Could you check a few things on this model? Use its own coordinates, in mm. A direction names the side the tool comes from. Give positions to 0.01 mm unless a question says otherwise; leave off trailing zeros. Order: outer loops, then holes, each group sorted by start corner. A loop starts at its lowest first (then second) coordinate and runs counter-clockwise, first axis right, second up. Notation, with made-up numbers: M -15.5,78.5 L 10.5,78.5 A9 ccw 10.5,94.5 Z; hole C -1.75,18.5 d7. An arc over 180 degrees is marked long. Use a Markdown table: item, result. Add a question column.
Item 1: Suppose I cut it at A-A on y = 5. Count the separate pieces of the cut face and the enclosed holes in it, plus the area to 3 significant figures.
Item 2: I'm going to push flat-ended pins straight in: pin 1 Ø1.9 at (x, y) = (20, 5) entering from -Z; pin 2 Ø3.5 at (x, y) = (20, 5) entering from +Z; pin 3 Ø3 at (y, z) = (12.5, 1.5) entering from +X; pin 4 Ø0.9 at (y, z) = (13.5, 1.5) entering from +X. Where does each tip first touch, or does it pass through?
Item 3: Suppose I cut it at B-B on x = 5. Write out the boundary of the cut face in (y, z), plus the area to 3 significant figures.
Item 4: If we mould it in two halves opening along X, with no side actions, what happens to faces 6 (the face through (1.141, 1.203, 2.524)), 7 (the face through (30, 5, 2)), 8 (the face through (5, 25, 2)), 9 (the face through (11.384, 2.338, 4.187))? For each: released by +X, released by -X, zero draft, split by the parting line, or undercut.
Item 5: If I drill on L1, parallel to X at y = 16.25, z = 3.4; L2, parallel to Y at x = 7.5, z = 3; L3, parallel to Y at x = 10, z = 3.9, over which ranges is the centre line in solid material (lowest first)? Write a range as from..to.
Item 6: Suppose I cut it at C-C on z = 1.75. Write out the boundary of the cut face in (x, y), plus the area to 3 significant figures.
Item 7: For faces 1 (the face through (22.5, 14, 2)), 2 (the face through (0.23, 5.77, 4.76)), 3 (the face through (21.3, 3.7, 3.35)), 4 (the face through (-3, 10, 2)), 5 (the face through (25.51, 9.77, 4.76)), which set-ups out of +Z, -Z, +X, -X, +Y, -Y let a thin tool reach every point of the face, with its end or its side?
from build123d import *

# Parameters (mm, degrees)
SKETCH2_W                       = 15
SKETCH2_H                       = 15
BOSS_EXTRUDE1_DEPTH             = 5
M3_CLEARANCE_HOLE1_OUTLINE_R    = 1.6
M3_CLEARANCE_HOLE1_DEPTH        = 5
CBORE_FOR_M3_SBHCS1_D           = 3.2
CBORE_FOR_M3_SBHCS1_CBORE_D     = 6
CBORE_FOR_M3_SBHCS1_CBORE_DEPTH = 1.65
CHAMFER1_SIZE                   = 8
FILLET1_R                       = 4
FILLET2_R                       = 2.5
FILLET3_R                       = 0.8


# Read off the part's stored shape, not the designer's step: M3 Clearance Hole1
with BuildPart() as part:
    # Sketch2 → Boss-Extrude1 (new body)
    with BuildSketch(Plane.XY):
        Polygon((0, 10), (0, 0), (30, 0), (30, 10), (22.5, 10), (7.5, 10), align=None)
        Polygon((-7.5, 10), (0, 10), (7.5, 10), (7.5, 25), (-7.5, 25), align=None)
        with Locations((15, 17.5)):
            Rectangle(SKETCH2_W, SKETCH2_H)
    extrude(amount=BOSS_EXTRUDE1_DEPTH)

    # M3 Clearance Hole1 outline → M3 Clearance Hole1 (cut)
    with BuildSketch(Plane.XY):
        with Locations((7.5, 17.5)):
            Circle(M3_CLEARANCE_HOLE1_OUTLINE_R)
        with Locations((-2.5, 17.5)):
            Circle(M3_CLEARANCE_HOLE1_OUTLINE_R)
        with Locations((25, 5)):
            Circle(M3_CLEARANCE_HOLE1_OUTLINE_R)
        with Locations((5, 5)):
            Circle(M3_CLEARANCE_HOLE1_OUTLINE_R)
    extrude(amount=M3_CLEARANCE_HOLE1_DEPTH, mode=Mode.SUBTRACT)

    # CBORE for M3 SBHCS1 (through all)
    with Locations(Plane.XY.offset(5)):
        with Locations((20, 5), (10, 5)):
            CounterBoreHole(CBORE_FOR_M3_SBHCS1_D / 2, CBORE_FOR_M3_SBHCS1_CBORE_D / 2, CBORE_FOR_M3_SBHCS1_CBORE_DEPTH)

    # Chamfer1
    chamfer1_edges = [part.edges().sort_by_distance(p)[0] for p in [
        (22.5, 25, 2.5),
    ]]
    chamfer(chamfer1_edges, length=CHAMFER1_SIZE)

    # Fillet1
    fillet1_edges = [part.edges().sort_by_distance(p)[0] for p in [
        (-7.5, 10, 2.5),
        (-7.5, 25, 2.5),
        (30, 10, 2.5),
        (30, 0, 2.5),
        (0, 0, 2.5),
        (14.5, 25, 2.5),
        (22.5, 17, 2.5),
    ]]
    fillet(fillet1_edges, radius=FILLET1_R)

    # Fillet2
    fillet2_edges = [part.edges().sort_by_distance(p)[0] for p in [
        (22.5, 10, 2.5),
        (0, 10, 2.5),
    ]]
    fillet(fillet2_edges, radius=FILLET2_R)

    # Fillet3
    fillet3_edges = [part.edges().sort_by_distance(p)[0] for p in [
        (14.37387948, 24.69551813, 5),
        (22.5, 13.921572875, 0),
        (22.5, 13.921572875, 5),
        (25.5, 10, 5),
        (25.5, 10, 0),
        (-3, 10, 5),
        (-3, 10, 0),
        (23.232233047, 10.732233047, 0),
        (23.232233047, 10.732233047, 5),
        (-0.732233047, 9.267766953, 0),
        (-0.732233047, 9.267766953, 5),
        (4.671572875, 25, 5),
        (4.671572875, 25, 0),
        (18.5, 21, 0),
        (30, 5, 0),
        (15, 0, 0),
        (0, 5.75, 0),
        (-7.5, 17.5, 0),
        (1.171572875, 1.171572875, 0),
        (28.828427125, 1.171572875, 0),
        (28.828427125, 8.828427125, 0),
        (-6.328427125, 11.171572875, 0),
        (-6.328427125, 23.828427125, 0),
        (22.19551813, 16.87387948, 0),
        (14.37387948, 24.69551813, 0),
        (18.5, 21, 5),
        (-7.5, 17.5, 5),
        (0, 5.75, 5),
        (15, 0, 5),
        (30, 5, 5),
        (1.171572875, 1.171572875, 5),
        (28.828427125, 1.171572875, 5),
        (28.828427125, 8.828427125, 5),
        (-6.328427125, 11.171572875, 5),
        (-6.328427125, 23.828427125, 5),
        (22.19551813, 16.87387948, 5),
    ]]
    fillet(fillet3_edges, radius=FILLET3_R)


solid = part.part
Findings below:
| question | item | result |
|---|---|---|
| 1 | separate pieces | 5 |
| 1 | enclosed holes | 0 |
| 1 | area | 76.2 mm^2 |
| 2 | pin 1 | passes through |
| 2 | pin 2 | stops at z = 3.35 |
| 2 | pin 3 | stops at x = 23 |
| 2 | pin 4 | stops at x = 22.5 |
| 3 | outline | M 0,0.8 A0.8 ccw 0.8,0 L 3.4,0 L 3.4,5 L 0.8,5 A0.8 ccw 0,4.2 Z; M 6.6,0 L 24.2,0 A0.8 ccw 25,0.8 L 25,4.2 A0.8 ccw 24.2,5 L 6.6,5 Z |
| 3 | area | 108 mm^2 |
| 4 | face 6 | released by -X |
| 4 | face 7 | released by +X |
| 4 | face 8 | zero draft |
| 4 | face 9 | undercut |
| 5 | L1 | x = -7.5..-3.5, -1.5..6.5, 8.5..22.4 |
| 5 | L2 | y = 0..15.9, 19.1..25 |
| 5 | L3 | y = 0..2, 8..25 |
| 6 | outline | M -7.5,14 A4 ccw -3.5,10 L -2.5,10 A2.5 cw 0,7.5 L 0,4 A4 ccw 4,0 L 26,0 A4 ccw 30,4 L 30,6 A4 ccw 26,10 L 25,10 A2.5 cw 22.5,12.5 L 22.5,15.34 A4 ccw 21.33,18.17 L 15.67,23.83 A4 ccw 12.84,25 L -3.5,25 A4 ccw -7.5,21 Z; hole C -2.5,17.5 d3.2; hole C 5,5 d3.2; hole C 7.5,17.5 d3.2; hole C 10,5 d3.2; hole C 20,5 d3.2; hole C 25,5 d3.2 |
| 6 | area | 655 mm^2 |
| 7 | face 1 | +Z, -Z, +X, +Y |
| 7 | face 2 | +Z, -X, -Y |
| 7 | face 3 | +Z |
| 7 | face 4 | +Z, -Z, -X, -Y |
| 7 | face 5 | +Z, +X, +Y |
